Could you check a few things on this drawing? It's one solid part, dimensions in mm from its lowest x, y, z. A direction names the side the tool comes from. Coordinates: 2 decimals unless noted, no trailing zeros. Write each loop counter-clockwise with the first axis right and the second up, starting at its lowest first coordinate (ties: lowest second). Pieces come first, ordered by that corner, then holes.
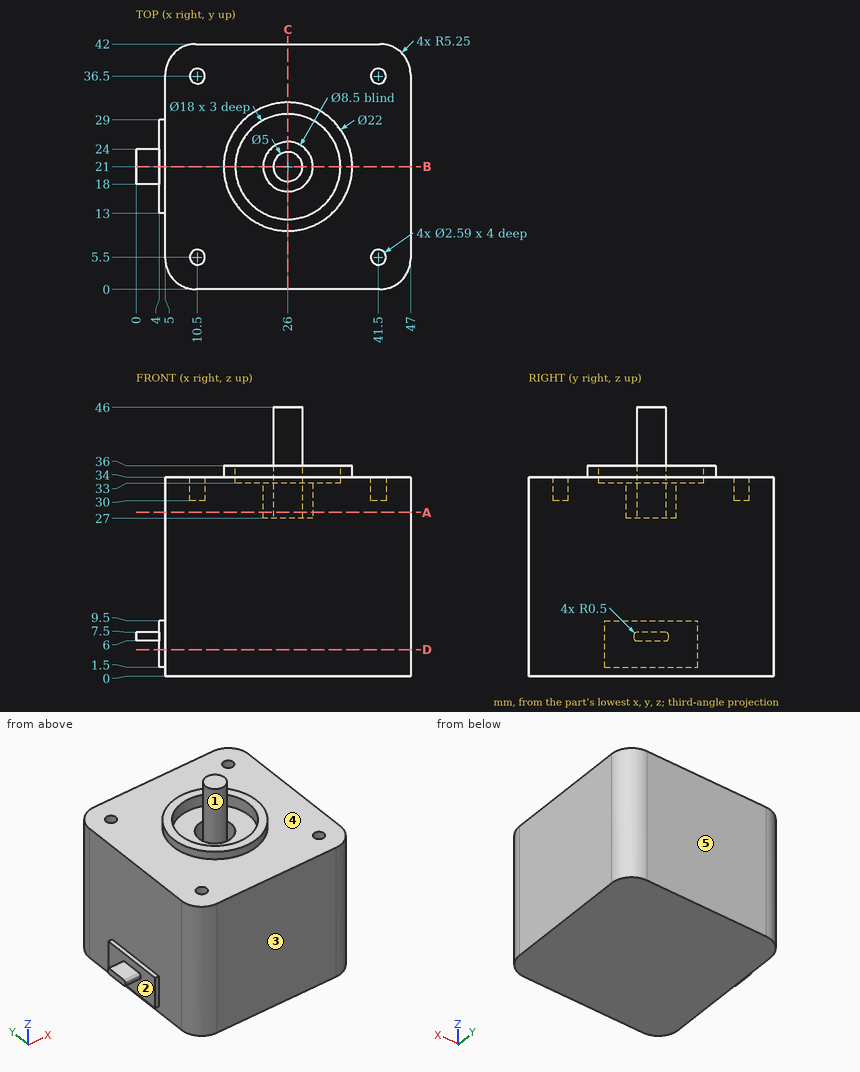
1) I need wall thicknesses on probe 1 along Y at (x, z) = (26, 29.7); probe 2 along Y at (x, z) = (41.5, 32.95) (3 decimals); probe 3 along Z at (x, y) = (20, 35). Which ranges of each line are inside material? Lowest first, please.
Values follow:
probe 1: y = 0 to 16.75, 18.5 to 23.5, 25.25 to 42
probe 2: y = 0 to 4.205, 6.795 to 35.205, 37.795 to 42
probe 3: z = 0 to 34
2) On a 3-axis mill with a long thin cutter (end or side, diameter ignored), from which of +Z, -Z, +X, -X, +Y, -Y can I reach the whole of each face in a straight line? I mean the marked faces 4 and 5. Say none if no direction works.
Values follow:
face 4: +Z
face 5: +Z, -Z, +X, -X, +Y
3) Imagine slicing it at D-D on z = 4.5. Please give me the cut outline in (x, y), then the cut area to 3 significant figures.
Values follow:
outline: (4, 13) - (5, 13) - (5, 5.25) arc R5.25 ccw to (10.25, 0) - (41.75, 0) arc R5.25 ccw to (47, 5.25) - (47, 36.75) arc R5.25 ccw to (41.75, 42) - (10.25, 42) arc R5.25 ccw to (5, 36.75) - (5, 29) - (4, 29) - close
area: 1,760 mm2
4) Imagine slicing it at B-B on y = 21. Please give me the cut outline in (x, z), then the cut area to 3 significant figures.
Values follow:
outline: (0, 6) - (4, 6) - (4, 1.5) - (5, 1.5) - (5, 0) - (47, 0) - (47, 34) - (37, 34) - (37, 36) - (35, 36) - (35, 33) - (30.25, 33) - (30.25, 27) - (28.5, 27) - (28.5, 46) - (23.5, 46) - (23.5, 27) - (21.75, 27) - (21.75, 33) - (17, 33) - (17, 36) - (15, 36) - (15, 34) - (5, 34) - (5, 9.5) - (4, 9.5) - (4, 7.5) - (0, 7.5) - close
area: 1,480 mm2
5) Imagine slicing it at A-A on z = 28. Please give me the cut outline in (x, y).
Values follow:
outline: (5, 5.25) arc R5.25 ccw to (10.25, 0) - (41.75, 0) arc R5.25 ccw to (47, 5.25) - (47, 36.75) arc R5.25 ccw to (41.75, 42) - (10.25, 42) arc R5.25 ccw to (5, 36.75) - close; circle Ø5 at (26, 21); hole circle Ø8.5 at (26, 21)
6) Imagine slicing it at C-C on x = 26. Please give me the cut outline in (y, z).
Values follow:
outline: (0, 0) - (42, 0) - (42, 34) - (32, 34) - (32, 36) - (30, 36) - (30, 33) - (25.25, 33) - (25.25, 27) - (23.5, 27) - (23.5, 46) - (18.5, 46) - (18.5, 27) - (16.75, 27) - (16.75, 33) - (12, 33) - (12, 36) - (10, 36) - (10, 34) - (0, 34) - close
7) We'd pull the mould along Y, two halves only. Please class the marked faces 1, 2 and 3: pulls with the +Y half, pulls with the -Y half, needs draft (parallel to the pull), parting line crosses it, or undercut.
Values follow:
face 1: undercut
face 2: needs draft
face 3: pulls with the -Y half
8) Will these pins go through, and if not, where does the flat tip stop? pin 1 (1.3 mm diameter, centred on x = 11, y = 5.5, fed in from +Z); pin 2 (10 mm diameter, centred on y = 25.5, z = 21, fed in from -X); pin 3 (0.6 mm diameter, centred on x = 2, z = 7, fed in from -Y).
Values follow:
pin 1: stops at z = 30
pin 2: stops at x = 5
pin 3: stops at y = 18
